```python
from build123d import *

# Parameters (mm, degrees)
BOSS_EXTRUDE1_DEPTH = 136
SKETCH5_R           = 5.5
LEFTWHEELS_DEPTH    = 5
RIGHTWHEELS_START   = -5
SKETCH6_R           = 5.5
RIGHTWHEELS_DEPTH   = 5
SKETCH7_R           = 1.9
FRONTHOLES_DEPTH    = 3
SKETCH8_R           = 1.85
TOPHOLES_DEPTH      = 3


with BuildPart() as part:
    # Sketch3 → Boss-Extrude1 (new body)
    with BuildSketch(Plane.XY):
        Polygon((-75, 23.5), (-105, 12), (-105, -12), (-75, -23.5), (75, -23.5), (105, -12), (105, 12), (75, 23.5), align=None)
    extrude(amount=BOSS_EXTRUDE1_DEPTH)

    # Sketch5 → LeftWheels (cut)
    with BuildSketch(Plane.XY.offset(136)):
        with Locations((78, 0)):
            Circle(SKETCH5_R)
        with Locations(Location((-78, 0, 0), (0, 0, 180))):
            Circle(SKETCH5_R)
    extrude(amount=-LEFTWHEELS_DEPTH, mode=Mode.SUBTRACT)

    # Sketch6 → RightWheels (cut)
    with BuildSketch(Plane(origin=(0, 0, 0), x_dir=(-1, 0, 0), z_dir=(0, 0, -1)).offset(RIGHTWHEELS_START)):
        with Locations((78, 0)):
            Circle(SKETCH6_R)
        with Locations(Location((-78, 0, 0), (0, 0, 180))):
            Circle(SKETCH6_R)
    extrude(amount=RIGHTWHEELS_DEPTH, mode=Mode.SUBTRACT)

    # Sketch7 → FrontHoles (cut)
    with BuildSketch(Plane(origin=(17.463066118, 45.555824655, 0), x_dir=(0.9337461173020496, -0.3579360116324526, 0), z_dir=(0.3579360116324526, 0.9337461173020496, 0))):
        with Locations(Location((77.683786351, -7, 0), (0, 0, 180))):
            Circle(SKETCH7_R)
        with Locations(Location((77.683786351, -22.25, 0), (0, 0, 180))):
            Circle(SKETCH7_R)
        with Locations(Location((77.683786351, -37.5, 0), (0, 0, 180))):
            Circle(SKETCH7_R)
        with Locations(Location((77.683786351, -52.75, 0), (0, 0, 180))):
            Circle(SKETCH7_R)
        with Locations(Location((77.683786351, -68, 0), (0, 0, 180))):
            Circle(SKETCH7_R)
        with Locations(Location((77.683786351, -83.25, 0), (0, 0, 180))):
            Circle(SKETCH7_R)
        with Locations(Location((77.683786351, -98.5, 0), (0, 0, 180))):
            Circle(SKETCH7_R)
        with Locations(Location((77.683786351, -113.75, 0), (0, 0, 180))):
            Circle(SKETCH7_R)
        with Locations(Location((77.683786351, -129, 0), (0, 0, 180))):
            Circle(SKETCH7_R)
    frontholes = extrude(amount=-FRONTHOLES_DEPTH, mode=Mode.SUBTRACT)

    # BackHoles: FrontHoles across plane
    add(frontholes.mirror(Plane(origin=(0, 0, 0), x_dir=(0, 0, 1), z_dir=(1, 0, 0))), mode=Mode.SUBTRACT)

    # Sketch8 → TopHoles (cut)
    with BuildSketch(Plane(origin=(0, 23.5, 0), x_dir=(1, 0, 0), z_dir=(0, 1, 0))):
        with Locations(Location((70.5, -7.25, 0), (0, 0, 180))):
            Circle(SKETCH8_R)
        with Locations(Location((70.5, -32, 0), (0, 0, 180))):
            Circle(SKETCH8_R)
        with Locations(Location((70.5, -50, 0), (0, 0, 180))):
            Circle(SKETCH8_R)
        with Locations(Location((70.5, -68, 0), (0, 0, 180))):
            Circle(SKETCH8_R)
        with Locations(Location((70.5, -86, 0), (0, 0, 180))):
            Circle(SKETCH8_R)
        with Locations(Location((70.5, -104, 0), (0, 0, 180))):
            Circle(SKETCH8_R)
        with Locations(Location((70.5, -128.75, 0), (0, 0, 180))):
            Circle(SKETCH8_R)
        with Locations((-70.5, -128.75)):
            Circle(SKETCH8_R)
        with Locations((-70.5, -104)):
            Circle(SKETCH8_R)
        with Locations((-70.5, -86)):
            Circle(SKETCH8_R)
        with Locations((-70.5, -68)):
            Circle(SKETCH8_R)
        with Locations((-70.5, -50)):
            Circle(SKETCH8_R)
        with Locations((-70.5, -32)):
            Circle(SKETCH8_R)
        with Locations((-70.5, -7.25)):
            Circle(SKETCH8_R)
    extrude(amount=-TOPHOLES_DEPTH, mode=Mode.SUBTRACT)


solid = part.part
```
The listing builds one solid part. Answer for the finished solid, in the listing's coordinates (mm). A direction names the side the tool comes from. Coordinates: 2 decimals unless noted, no trailing zeros. Loops run counter-clockwise (first coordinate to the right, second up) from the corner with the lowest first, then second, coordinate; pieces in that order, holes last. Notation, with made-up numbers: (83, -34) -> (129, -34) arc R34 cw to (129, 4) -> close; hole circle Ø3 at (-8, 1.25). An arc over 180 degrees is marked (long way). Use one line per item in the form item = value. Start each with the question number.
Item 1: The part is cut by section B-B on z = 60. Determine the outline of the cut face in (x, y).
Item 2: A tool of negligible diameter and unlimited length cuts with its end or side. For faces 5 (the face through (-89.855, 16.222, 50.895)), 6 (the face through (-72.505, 0.242, 2.535)), from which of +Z, -Z, +X, -X, +Y, -Y can it reach the whole face along a straight path? Write none if from no direction.
Item 3: Consider L1, parallel to Y at x = -96, z = 22.5; L2, parallel to Y at x = -87, z = 49.5. Determine where each line is inside the solid, lowest interval first. Write a range as [from, to].
Item 4: The part is cut by section A-A on x = 78. Determine the outline of the cut face in (y, z).
Item 5: Flat-ended cylindrical pins translate along their axes: pin 1 Ø3 at (x, z) = (-70.5, 104) entering from +Y; pin 2 Ø5 at (x, z) = (83.5, 28) entering from +Y; pin 3 Ø8 at (x, z) = (79.5, 95) entering from -Y. Find the tip coordinate at first contact, or state that the pin passes through.
Item 6: The mould has two halves that part along X. Classify faces 1 (the face through (89.855, 16.222, 66.145)), 2 (the face through (-86.457, 19.108, 67.048)), 3 (the face through (-89.855, 16.222, 111.895)), 4 (the face through (1, 23.5, 67)): released by +X, released by -X, zero draft, split by the parting line, or undercut.
Answer key:
q1.outline = (-105, -12) -> (-75, -23.5) -> (75, -23.5) -> (105, -12) -> (105, 12) -> (75, 23.5) -> (-75, 23.5) -> (-105, 12) -> close
q2.face_5 = none
q2.face_6 = -Z
q3.L1 = [-15.45, 15.45]
q3.L2 = [-18.9, 18.9]
q4.outline = (-22.35, 0) -> (-5.5, 0) -> (-5.5, 5) -> (5.5, 5) -> (5.5, 0) -> (22.35, 0) -> (22.35, 136) -> (5.5, 136) -> (5.5, 131) -> (-5.5, 131) -> (-5.5, 136) -> (-22.35, 136) -> close
q5.pin_1 = 20.5
q5.pin_2 = 21.2
q5.pin_3 = -23.31
q6.face_1 = undercut
q6.face_2 = released by -X
q6.face_3 = undercut
q6.face_4 = zero draft
